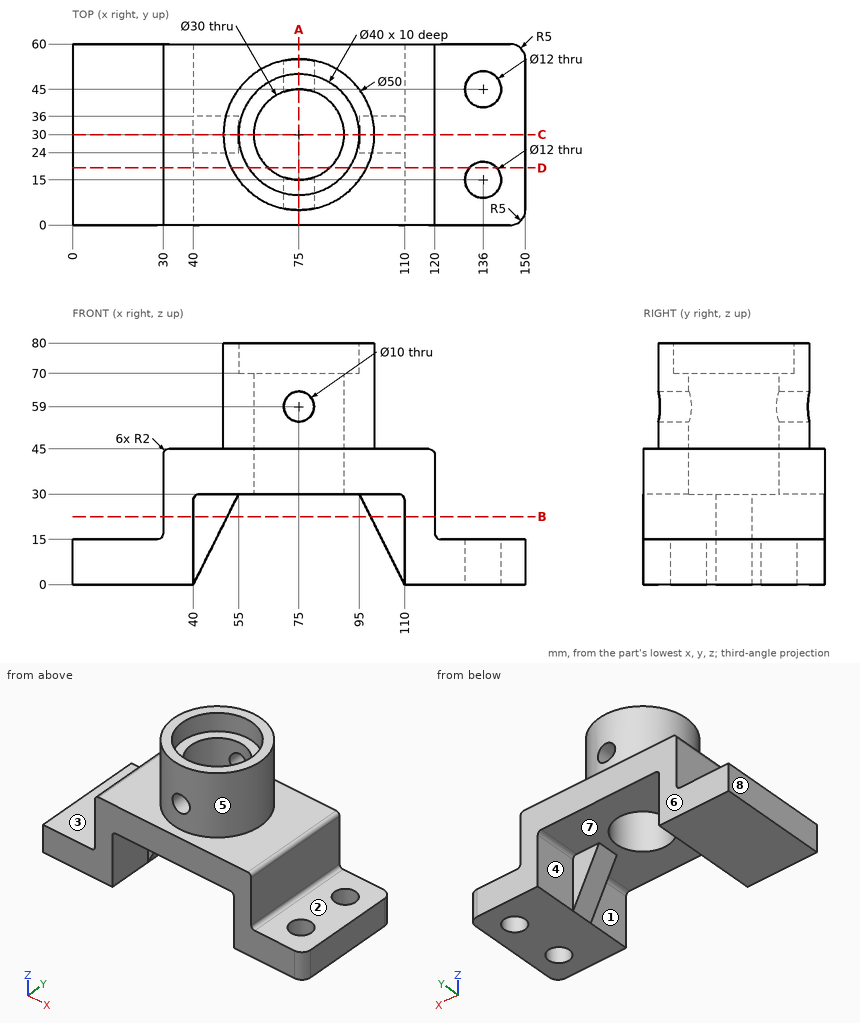
Print and shaded views of the part. All mm, measured from the part's lowest x, y and z. A direction names the side the tool comes from. Give positions to 0.01 mm unless a question says otherwise; leave off trailing zeros. Order: outer loops, then holes, each group sorted by start corner. A loop starts at its lowest first (then second) coordinate and runs counter-clockwise, first axis right, second up. Notation, with made-up numbers: (-36, 70.5) - (11, 70.5) arc R14 ccw to (11, 83.5) - close; hole circle Ø3 at (-26.75, 3.25). An arc over 180 degrees is marked (long way). Use a Markdown table: item, result.
1) Saw through at D-D on y = 19. Count the separate pieces of the cut face and the enclosed holes in it, plus the area to 3 significant figures.
Checked values:
| item | result |
|---|---|
| separate pieces | 3 |
| enclosed holes | 0 |
| area | 3,140 mm² |
2) Probe L1, parallel to X at y = 15, z = 10; L2, parallel to Z at x = 75, y = 12; L3, parallel to Y at x = 136, z = 11. List the from-to ranges inside material, lowest first. Write a range as from..to.
Checked values:
| item | result |
|---|---|
| L1 | 0..40, 110..130, 142..150 |
| L2 | 30..54, 64..70 |
| L3 | 0..9, 21..39, 51..60 |
3) Saw through at C-C on y = 30. List the corners of the cut face in (x, z).
Checked values:
| item | result |
|---|---|
| outline | (0, 0) - (40, 0) - (55, 30) - (60, 30) - (60, 70) - (55, 70) - (55, 80) - (50, 80) - (50, 45) - (32, 45) arc R2 ccw to (30, 43) - (30, 17) arc R2 cw to (28, 15) - (0, 15) - close; (90, 30) - (95, 30) - (110, 0) - (150, 0) - (150, 15) - (122, 15) arc R2 cw to (120, 17) - (120, 43) arc R2 ccw to (118, 45) - (100, 45) - (100, 80) - (95, 80) - (95, 70) - (90, 70) - close |
4) 3-axis set-ups, long thin cutter, end or side, ignore diameter. For the marked faces 1, 2, 3, 4 and 5: which of +Z, -Z, +X, -X, +Y, -Y reach the whole face in a straight line?
Checked values:
| item | result |
|---|---|
| face 1 | -Z, -Y |
| face 2 | +Z, +X, +Y, -Y |
| face 3 | +Z, -X, +Y, -Y |
| face 4 | -Z, +Y |
| face 5 | +Z |
5) Saw through at B-B on z = 22.5. List the corners of the cut face in (x, y).
Checked values:
| item | result |
|---|---|
| outline | (30, 0) - (40, 0) - (40, 24) - (51.25, 24) - (51.25, 36) - (40, 36) - (40, 60) - (30, 60) - close; (98.75, 24) - (110, 24) - (110, 0) - (120, 0) - (120, 60) - (110, 60) - (110, 36) - (98.75, 36) - close |
6) Flat gauge pins, fed straight in: P1, Ø16.5, axis at x = 45.5, z = 11, coming from the -Y side; P2, Ø12, axis at x = 46.5, z = 11, coming from the +Y side; P3, Ø20, axis at x = 79, y = 23, coming from the +Z side; P4, Ø4.5, axis at x = 102.5, z = 18.5, coming from the -Y side. Where does each tip first touch, or does it go through?
Checked values:
| item | result |
|---|---|
| P1 | y = 0 |
| P2 | y = 36 |
| P3 | z = 70 |
| P4 | y = 24 |
7) Two-plate mould, pull along X, no slides. Class the marked faces 6, 7 and 8: +X half, -X half, draft (parallel to the pull), parting line (faces both ways), or undercut.
Checked values:
| item | result |
|---|---|
| face 6 | draft |
| face 7 | undercut |
| face 8 | -X half |
8) Saw through at A-A on x = 75. List the corners of the cut face in (y, z).
Checked values:
| item | result |
|---|---|
| outline | (0, 30) - (15, 30) - (15, 54) - (5, 54) - (5, 45) - (0, 45) - close; (5, 64) - (15, 64) - (15, 70) - (10, 70) - (10, 80) - (5, 80) - close; (45, 30) - (60, 30) - (60, 45) - (55, 45) - (55, 54) - (45, 54) - close; (45, 64) - (55, 64) - (55, 80) - (50, 80) - (50, 70) - (45, 70) - close |
